```python
from build123d import *

# Parameters (mm, degrees)
BOSS_EXTRUDE1_DEPTH        = 10
BOSS_EXTRUDE2_DEPTH        = 15
F_20_0_20_DIAMETER_HOLE1_D = 20
F_12_0_12_DIAMETER_HOLE1_D = 12
FILLET1_R                  = 5


with BuildPart() as part:
    # Sketch2 → Boss-Extrude1 (new body)
    with BuildSketch(Plane(origin=(0, 0, 0), x_dir=(1, 0, 0), z_dir=(0, 1, 0))):
        with BuildLine():
            Line((0, 0), (110, 0))
            Line((110, 0), (110, -15))
            ThreePointArc((110, -15), (105.270148503, -28.695601287), (93.096662434, -36.553541647))
            Line((93.096662434, -36.553541647), (24.767095445, -53.323563036))
            ThreePointArc((24.767095445, -53.323563036), (7.657834649, -49.637565074), (0, -33.9))
            Line((0, -33.9), (0, 0))
        make_face()
    extrude(amount=BOSS_EXTRUDE1_DEPTH)

    # Sketch4 → Boss-Extrude2 (add)
    with BuildSketch(Plane(origin=(0, 0, 0), x_dir=(-1, 0, 0), z_dir=(0, 0, -1))):
        with BuildLine():
            Line((-110, 10), (-40, 10))
            Line((-40, 10), (-40, 26.4))
            ThreePointArc((-40, 26.4), (-45.795793145, 38.24409457), (-58.70434349, 40.935399523))
            Line((-58.70434349, 40.935399523), (-100.345866401, 30.323066228))
            ThreePointArc((-100.345866401, 30.323066228), (-107.302721394, 25.766620463), (-110, 17.9))
            Line((-110, 17.9), (-110, 10))
        make_face()
    extrude(amount=-BOSS_EXTRUDE2_DEPTH)

    # Ø20.0 (20) Diameter Hole1 (through all)
    with Locations(Plane(origin=(20, 10, 33.9), x_dir=(0, 0, 1), z_dir=(0, 1, 0))):
        with Locations((0, 0)):
            Hole(F_20_0_20_DIAMETER_HOLE1_D / 2)

    # Ø12.0 (12) Diameter Hole1 (through all)
    with Locations(Plane(origin=(55, 26.4, 15), x_dir=(1, 0, 0), z_dir=(0, 0, 1))):
        with Locations((0, 0)):
            Hole(F_12_0_12_DIAMETER_HOLE1_D / 2)

    # Fillet1
    fillet1_edges = [part.edges().sort_by_distance(p)[0] for p in [
        (75, 10, 15),
    ]]
    fillet(fillet1_edges, radius=FILLET1_R)


solid = part.part
```
Can you work these out from the model? Positions are in its coordinate system, mm. A direction names the side the tool comes from. Round coordinates to 2 decimals unless told otherwise and drop trailing zeros. Loops run counter-clockwise (first coordinate to the right, second up) from the corner with the lowest first, then second, coordinate; pieces in that order, holes last. Notation, with made-up numbers: (-1, 73) -> (45, 73) arc R13 cw to (45, 84) -> close; hole circle Ø10 at (18, 7.5). An arc over 180 degrees is marked (long way). One line per item, written item: value. Start each with the question number.
1. If I drill on probe 1 along Y at (x, z) = (55, 5.25); probe 2 along X at (y, z) = (26, 7); probe 3 along X at (y, z) = (16, 11.5), over which ranges is the centre line in solid material (lowest first)?
2. For faces 5 (the flat face through (43, 10, 27)), 6 (the flat face through (59.41, 4.93, 44.82)), 7 (the flat face through (75, 25, 15)), 8 (the flat face through (40, 18, 8)), 9 (the flat face through (68, 16, 0)), which set-ups out of +Z, -Z, +X, -X, +Y, -Y let a thin tool reach every point of the face, with its end or its side?
3. If we section it at C-C, the plane z = 10: Write out the boundary of the cut face in (x, y), then the cut area to 3 significant figures.
4. If we section it at B-B, the plane y = 7: Write out the boundary of the cut face in (x, z), then the cut area to 3 significant figures.
5. If we section it at D-D, the plane z = 28.5: Write out the boundary of the cut face in (x, y).
6. For pin 1 (8 mm diameter, centred on x = 79.5, y = 28.5, fed in from +Z); pin 2 (8 mm diameter, centred on x = 93.5, y = 15, fed in from +Z); pin 3 (10 mm diameter, centred on x = 98, z = 22.5, fed in from +Y), each with a flat end and sliding along its axis, tell me the tip position at first contact or that it passes through.
7. If we section it at A-A, the plane x = 20: Write out the boundary of the cut face in (y, z), then the cut area to 3 significant figures.
8. If we mould it in two halves opening along Y, with no side actions, what happens to faces 1 (the flat face through (56, 0, 21)), 2 (the flat face through (110, 9, 7)), 3 (the cylindrical face through (107.2, 25.9, 7.4)), 4 (the cylindrical face through (60.994, 26.664, 7.395))? For each: pulls with the +Y half, pulls with the -Y half, needs draft (parallel to the pull), parting line crosses it, or undercut.
Calculated:
1. probe 1: y = 0 to 20.4, 32.4 to 41.4
1. probe 2: x = 40 to 49.01, 60.99 to 107.12
1. probe 3: x = 40 to 110
2. face 5: +Z, -X, +Y
2. face 6: +Z, +X, +Y, -Y
2. face 7: +Z, +X, -X, +Y
2. face 8: +Z, -Z, -X, +Y
2. face 9: -Z, +X, -X, +Y, -Y
3. outline: (0, 0) -> (110, 0) -> (110, 17.9) arc R12.82 ccw to (100.35, 30.32) -> (58.7, 40.94) arc R15 ccw to (40, 26.4) -> (40, 10) -> (0, 10) -> close; hole circle Ø12 at (55, 26.4)
3. area: 2,760 mm²
4. outline: (0, 0) -> (110, 0) -> (110, 15) arc R22.19 ccw to (93.1, 36.55) -> (24.77, 53.32) arc R20 ccw to (0, 33.9) -> close; hole circle Ø20 at (20, 33.9)
4. area: 4,530 mm²
5. outline: (0, 0) -> (11.58, 0) -> (11.58, 10) -> (0, 10) -> close; (28.42, 0) -> (105.42, 0) -> (105.42, 10) -> (28.42, 10) -> close
6. pin 1: stops at z = 15
6. pin 2: stops at z = 17
6. pin 3: stops at y = 10.67
7. outline: (0, 0) -> (10, 0) -> (10, 23.9) -> (0, 23.9) -> close; (0, 43.9) -> (10, 43.9) -> (10, 53.9) -> (0, 53.9) -> close
7. area: 339 mm²
8. face 1: pulls with the -Y half
8. face 2: needs draft
8. face 3: pulls with the +Y half
8. face 4: undercut
